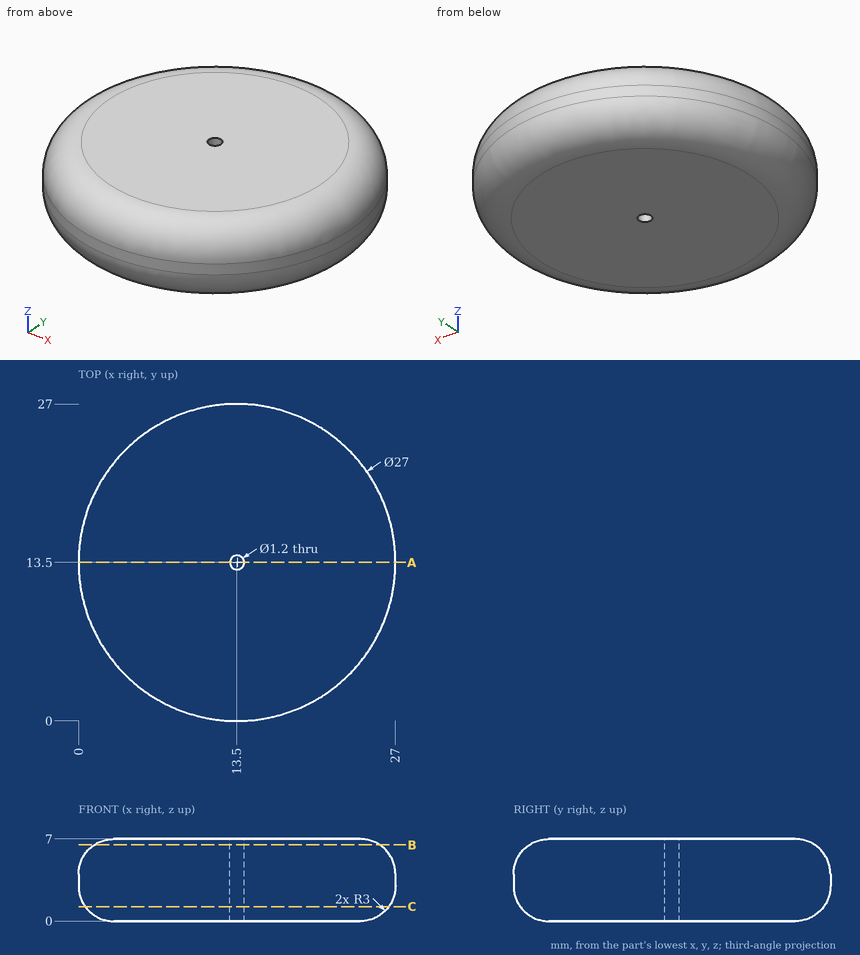
Verification items for this drawing (mm, ordinates from the low corner). Coordinates: 2 decimals unless noted, no trailing zeros. Order: outer loops, then holes, each group sorted by start corner. A loop starts at its lowest first (then second) coordinate and runs counter-clockwise, first axis right, second up. Notation, with made-up numbers: (49.5, 57) - (79.5, 57) arc R20 ccw to (79.5, 76) - close; hole circle Ø9 at (78.5, 70.25). An arc over 180 degrees is marked (long way). Answer in a Markdown table with one row per item. Add a question column.
1. Gauge pin test, flat ends, axial feed: pin 1 Ø1.9 at (x, y) = (13.5, 13.5) entering from +Z; pin 2 Ø2 at (x, z) = (16, 2) entering from -Y; pin 3 Ø4 at (x, z) = (3.5, 2.5) entering from +Y; pin 4 Ø2 at (x, y) = (7.5, 24) entering from +Z. Record the tip position at first contact, or that the pin passes through.
2. Section check A-A (y = 13.5). Enter the section's corners in (x, z).
3. Section check B-B (z = 6.5). Enter the section's corners in (x, y), plus the area to 3 significant figures.
4. Material ranges on L1, parallel to Y at x = 13.5, z = 3.75; L2, parallel to Y at x = 13.5, z = 1.5; L3, parallel to Z at x = 24.75, y = 13, recorded low to high. Write a range as [from, to].
5. Section check C-C (z = 1.25). Enter the section's corners in (x, y), plus the area to 3 significant figures.
Data:
| question | item | result |
|---|---|---|
| 1 | pin 1 | stops at z = 7 |
| 1 | pin 2 | stops at y = 0.13 |
| 1 | pin 3 | stops at y = 24.35 |
| 1 | pin 4 | stops at z = 6.94 |
| 2 | outline | (0, 3) arc R3 ccw to (3, 0) - (12.9, 0) - (12.9, 7) - (3, 7) arc R3 ccw to (0, 4) - close; (14.1, 0) - (24, 0) arc R3 ccw to (27, 3) - (27, 4) arc R3 ccw to (24, 7) - (14.1, 7) - close |
| 3 | outline | circle Ø24.32 at (13.5, 13.5); hole circle Ø1.2 at (13.5, 13.5) |
| 3 | area | 463 mm² |
| 4 | L1 | y = [0, 12.9], [14.1, 27] |
| 4 | L2 | y = [0.4, 12.9], [14.1, 26.6] |
| 4 | L3 | z = [0.1, 6.9] |
| 5 | outline | circle Ø25.87 at (13.5, 13.5); hole circle Ø1.2 at (13.5, 13.5) |
| 5 | area | 525 mm² |
